from build123d import *

# Parameters (mm, degrees)
F1_DEPTH = 1.016
F3_D     = 3.81
F4_R     = 1.905
F5_DEPTH = 1.27
F6_R     = 1.26999


# Not quite as in the source:
# - a fillet or chamfer is up to 0.001 mm smaller than in the source, because OpenCascade refuses the exact size


with BuildPart() as f1:
    # F0 (on Top) → F1 (new body)
    with BuildSketch(Plane.XY):
        with BuildLine():
            ThreePointArc((3.81, -3.81), (6.5040768363, -2.6940768363), (7.62, 0))
            ThreePointArc((7.62, 0), (6.5040768363, 2.6940768363), (3.81, 3.81))
            ThreePointArc((3.81, 3.81), (1.1159231637, 2.6940768363), (0, 0))
            ThreePointArc((0, 0), (1.1159231637, -2.6940768363), (3.81, -3.81))
        make_face()
        with BuildLine():
            ThreePointArc((0, 0), (1.1159231637, 2.6940768363), (3.81, 3.81))
            Line((3.81, 3.81), (-3.81, 3.81))
            ThreePointArc((-3.81, 3.81), (-1.1159231637, 2.6940768363), (0, 0))
        make_face()
        with BuildLine():
            Line((-3.81, -3.81), (3.81, -3.81))
            ThreePointArc((3.81, -3.81), (1.1159231637, -2.6940768363), (0, 0))
            ThreePointArc((0, 0), (-1.1159231637, -2.6940768363), (-3.81, -3.81))
        make_face()
        with BuildLine():
            ThreePointArc((-3.81, -3.81), (-1.1159231637, -2.6940768363), (0, 0))
            ThreePointArc((0, 0), (-1.1159231637, 2.6940768363), (-3.81, 3.81))
            ThreePointArc((-3.81, 3.81), (-7.62, 0), (-3.81, -3.81))
        make_face()
    extrude(amount=F1_DEPTH)

    # F3 (through all)
    with Locations(Plane.XY.offset(1.016)):
        with Locations((-3.81, 0)):
            Hole(F3_D / 2)

    # F4 (on face) → F5 (join)
    with BuildSketch(Plane(origin=(0, 0, 0), x_dir=(1, 0, 0), z_dir=(0, 0, -1))):
        with Locations((3.81, 0)):
            Circle(F4_R)
    extrude(amount=F5_DEPTH)

    # F6 (radius 1.27 in the source; OpenCascade refuses exactly that, so slightly less here)
    f6_edges = [f1.edges().sort_by_distance(p)[0] for p in [
        (1.905, 0, -1.27),
    ]]
    fillet(f6_edges, radius=F6_R)


solid = f1.part
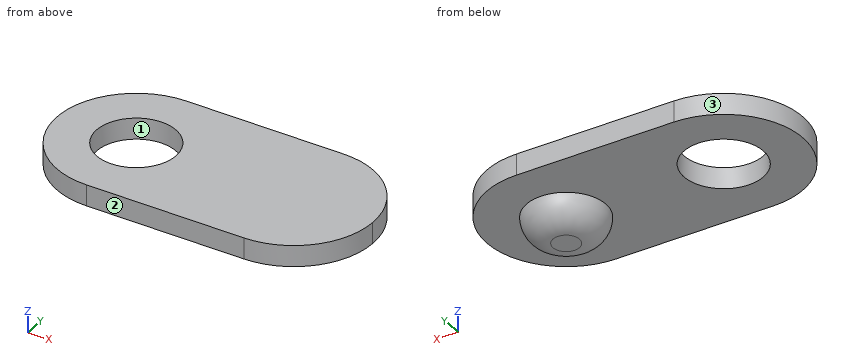
The model under review builds one solid part; all positions refer to its coordinate system, in mm. Face numbers are marked on the shaded views. Coordinates: 2 decimals unless noted, no trailing zeros. Loops run counter-clockwise (first coordinate to the right, second up) from the corner with the lowest first, then second, coordinate; pieces in that order, holes last. Notation, with made-up numbers: M 39,19.5 L 84,19.5 A28 ccw 84,56.5 Z; hole C 12,13.25 d11. An arc over 180 degrees is marked long. Put each result on its own line as item: value. Start each with the question number.
Q1. Add section A-A (z = 0.35). Write out the cut boundary in (x, y) (3 decimals).
Q2. Wall thickness on line 1 (Y direction, x = -3.81, z = 0.65) (3 decimals); line 2 (Z direction, x = -6.25, y = -1.75); line 3 (Y direction, x = 5.5, z = 0.7): over which ranges is each line inside the solid? List them lowest first.
Q3. Add section B-B (x = 0.5). Write out the cut boundary in (y, z).
Q4. The part is to be moulded in two halves that separate along X. For the marked faces 1, 2 and 3, say which applies: +X half, -X half, draft (parallel to the pull), parting line (faces both ways), or undercut.
Q5. Add section C-C (y = 3). Write out the cut boundary in (x, z).
Answers:
1. outline: M -3.81,-3.81 L 3.81,-3.81 A3.81 ccw 3.81,3.81 L -3.81,3.81 A3.81 ccw Z; hole C -3.81,0 d3.81
2. line 1: y = -3.81 to -1.905, 1.905 to 3.81
2. line 2: z = 0 to 1.02
2. line 3: y = -3.41 to 3.41
3. outline: M -3.81,0 L 3.81,0 L 3.81,1.02 L -3.81,1.02 Z
4. face 1: undercut
4. face 2: draft
4. face 3: -X half
5. outline: M -6.16,0 L 6.16,0 L 6.16,1.02 L -6.16,1.02 Z
